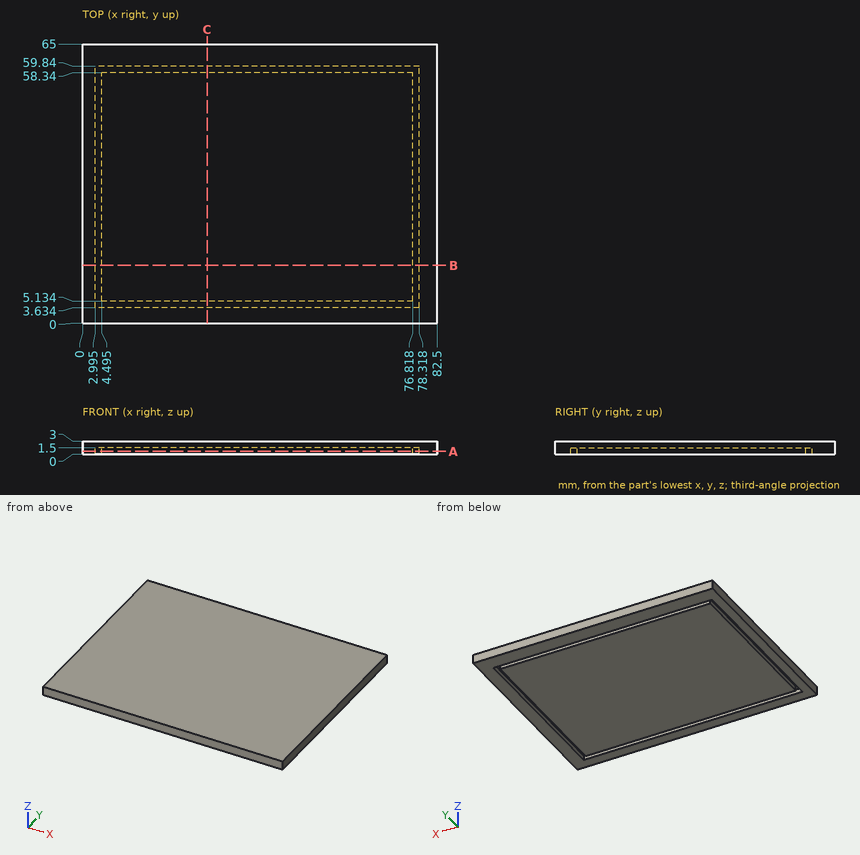
The figure shows three views and two pictorial views of one solid part (mm, origin at its lowest corner). Answer the questions. Coordinates: 2 decimals unless noted, no trailing zeros. Loops run counter-clockwise (first coordinate to the right, second up) from the corner with the lowest first, then second, coordinate; pieces in that order, holes last. Notation, with made-up numbers: (19, 8.5) - (28, 8.5) arc R35 cw to (28, 41.5) - close; hole circle Ø2 at (-7.5, -27). An arc over 180 degrees is marked (long way). Answer in a Markdown table with one row per item.
Q1. Find section A-A on z = 0.65. Write down the section's boundary in (x, y) (1 decimal).
Here are the results:
| item | result |
|---|---|
| outline | (0, 0) - (82.5, 0) - (82.5, 65) - (0, 65) - close; (4.5, 5.1) - (76.8, 5.1) - (76.8, 58.3) - (4.5, 58.3) - close; hole (3, 3.6) - (78.3, 3.6) - (78.3, 59.8) - (3, 59.8) - close |
Q2. Straight lines are drawn through the part: line 1 along Y through (x, z) = (67.5, 0.6); line 2 along X through (y, z) = (46, 0.5) (1 decimal); line 3 along Z through (x, y) = (66.5, 4). For each, find the intervals that lie inside material, in ascending order. Write a range as [from, to].
Here are the results:
| item | result |
|---|---|
| line 1 | y = [0, 3.63], [5.13, 58.34], [59.84, 65] |
| line 2 | x = [0, 3], [4.5, 76.8], [78.3, 82.5] |
| line 3 | z = [1.5, 3] |
Q3. Find section C-C on x = 29. Write down the section's boundary in (y, z).
Here are the results:
| item | result |
|---|---|
| outline | (0, 0) - (3.63, 0) - (3.63, 1.5) - (5.13, 1.5) - (5.13, 0) - (58.34, 0) - (58.34, 1.5) - (59.84, 1.5) - (59.84, 0) - (65, 0) - (65, 3) - (0, 3) - close |
Q4. Find section B-B on y = 13.5. Write down the section's boundary in (x, z) (1 decimal), plus the area to 3 significant figures.
Here are the results:
| item | result |
|---|---|
| outline | (0, 0) - (3, 0) - (3, 1.5) - (4.5, 1.5) - (4.5, 0) - (76.8, 0) - (76.8, 1.5) - (78.3, 1.5) - (78.3, 0) - (82.5, 0) - (82.5, 3) - (0, 3) - close |
| area | 243 mm^2 |
